Input: part model. Units: mm. Frame: model coordinates. Face numbers are marked on the shaded views. A direction names the side the tool comes from. Round coordinates to 2 decimals unless told otherwise and drop trailing zeros. Order: outer loops, then holes, each group sorted by start corner. A loop starts at its lowest first (then second) coordinate and runs counter-clockwise, first axis right, second up. Notation, with made-up numbers: (-39.5, 52.5) -> (-12.5, 52.5) arc R27 ccw to (-12.5, 68.5) -> close; hole circle Ø4 at (30.5, 82). An arc over 180 degrees is marked (long way). Use a Markdown table: item, result.
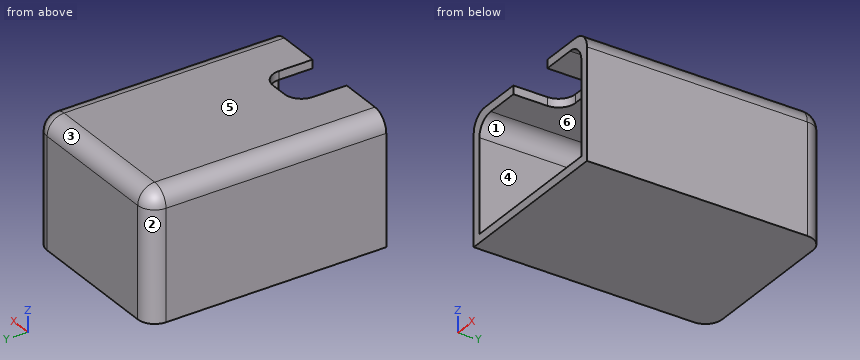
from build123d import *

# Parameters (mm, degrees)
F0_W     = 20
F0_H     = 15
F1_DEPTH = 28
F2_T     = -1
F3_R     = 2
F4_R     = 2
F5_R     = 2
F7_DEPTH = 1
F8_R     = 2


with BuildPart() as f1:
    # F0 (on Front) → F1 (new body)
    with BuildSketch(Plane.XZ):
        Rectangle(F0_W, F0_H)
    extrude(amount=F1_DEPTH)

    # F2
    f2_openings = [f1.faces().sort_by_distance(p)[0] for p in [
        (0, -28, 0),
    ]]
    offset(amount=F2_T, openings=f2_openings)

    # F3
    f3_edges = [f1.edges().sort_by_distance(p)[0] for p in [
        (-9, -14.5, 6.5),
        (9, -14.5, 6.5),
    ]]
    fillet(f3_edges, radius=F3_R)

    # F4
    f4_edges = [f1.edges().sort_by_distance(p)[0] for p in [
        (10, -14, 7.5),
        (-10, -14, 7.5),
    ]]
    fillet(f4_edges, radius=F4_R)

    # F5
    f5_edges = [f1.edges().sort_by_distance(p)[0] for p in [
        (0, 0, 7.5),
        (10, 0, -1),
        (-10, 0, -1),
    ]]
    fillet(f5_edges, radius=F5_R)

    # F6 (on face) → F7 (cut, through all)
    with BuildSketch(Plane.XY.offset(7.5)):
        Polygon((3, -28), (3, -22), (-3, -22), (-3, -28), (0, -28), align=None)
    extrude(amount=-F7_DEPTH, mode=Mode.SUBTRACT)

    # F8
    f8_edges = [f1.edges().sort_by_distance(p)[0] for p in [
        (-3, -22, 7),
        (3, -22, 7),
    ]]
    fillet(f8_edges, radius=F8_R)


solid = f1.part
1) Line query: L1, parallel to Z at x = 1, y = -12.75; L2, parallel to X at y = -6, z = 3.25; L3, parallel to Y at x = -3, z = 0.5. Output: solid intervals per line, ascending. Write a range as [from, to].
Results found:
| item | result |
|---|---|
| L1 | z = [-7.5, -6.5], [6.5, 7.5] |
| L2 | x = [-10, -9], [9, 10] |
| L3 | y = [-1, 0] |
2) Set-up query: the marked faces 5 and 6. Return all of +Z, -Z, +X, -X, +Y, -Y with unobstructed straight access to the full face (end or side cutting, diameter ignored); none if empty.
Results found:
| item | result |
|---|---|
| face 5 | +Z, +X, -X, +Y, -Y |
| face 6 | -Y |
3) Pin query (flat end, axial travel): pin 1 Ø6 at (x, z) = (-7.5, 4) entering from -Y; pin 2 Ø1.1 at (y, z) = (-26.5, 7) entering from +X; pin 3 Ø0.5 at (y, z) = (-26.5, 7) entering from -X; pin 4 Ø6.5 at (x, z) = (1.5, -3) entering from -Y. Return the tip coordinate at first contact, or that it passes through.
Results found:
| item | result |
|---|---|
| pin 1 | stops at y = -28 |
| pin 2 | stops at x = 9.76 |
| pin 3 | stops at x = -9.56 |
| pin 4 | stops at y = -1 |
4) Cut plane A-A on y = -4. Return loops of the section in (x, z).
Results found:
| item | result |
|---|---|
| outline | (-10, -7.5) -> (10, -7.5) -> (10, 5.5) arc R2 ccw to (8, 7.5) -> (-8, 7.5) arc R2 ccw to (-10, 5.5) -> close; hole (-9, -6.5) -> (9, -6.5) -> (9, 4.5) arc R2 ccw to (7, 6.5) -> (-7, 6.5) arc R2 ccw to (-9, 4.5) -> close |
5) Cut plane D-D on y = -25. Return loops of the section in (x, z).
Results found:
| item | result |
|---|---|
| outline | (-10, -7.5) -> (10, -7.5) -> (10, 5.5) arc R2 ccw to (8, 7.5) -> (3, 7.5) -> (3, 6.5) -> (7, 6.5) arc R2 cw to (9, 4.5) -> (9, -6.5) -> (-9, -6.5) -> (-9, 4.5) arc R2 cw to (-7, 6.5) -> (-3, 6.5) -> (-3, 7.5) -> (-8, 7.5) arc R2 ccw to (-10, 5.5) -> close |
6) Cut plane C-C on z = -4.5. Return loops of the section in (x, y), and give its area (3 significant figures).
Results found:
| item | result |
|---|---|
| outline | (-10, -28) -> (-9, -28) -> (-9, -1) -> (9, -1) -> (9, -28) -> (10, -28) -> (10, -2) arc R2 ccw to (8, 0) -> (-8, 0) arc R2 ccw to (-10, -2) -> close |
| area | 72.3 mm² |
7) Pull-direction query (X, two-part tool) for the marked faces 1, 2, 3 and 4; classes: +X half, -X half, draft (parallel to the pull), parting line (faces both ways), or undercut.
Results found:
| item | result |
|---|---|
| face 1 | undercut |
| face 2 | -X half |
| face 3 | draft |
| face 4 | undercut |
8) Cut plane B-B on x = 5.75. Return loops of the section in (y, z), and give its area (3 significant figures).
Results found:
| item | result |
|---|---|
| outline | (-28, -7.5) -> (0, -7.5) -> (0, 5.5) arc R2 ccw to (-2, 7.5) -> (-28, 7.5) -> (-28, 6.5) -> (-1, 6.5) -> (-1, -6.5) -> (-28, -6.5) -> close |
| area | 68.1 mm² |
